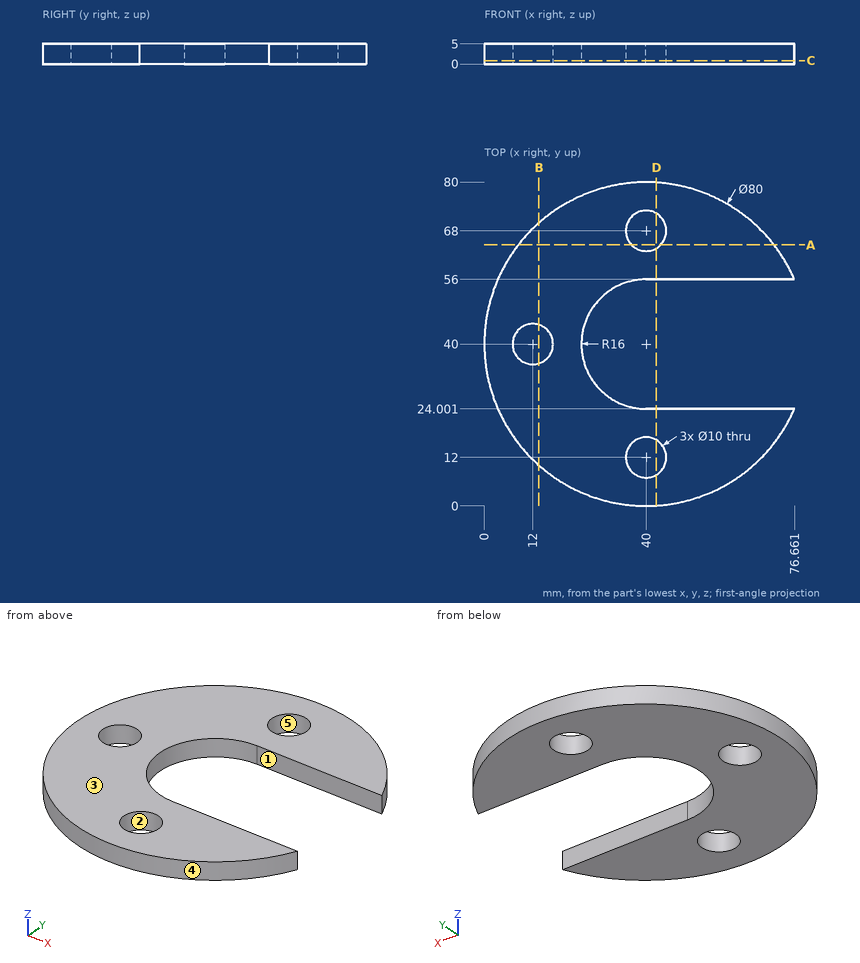
Design review of the part shown in the three views and the two pictorial views. Dimensions are in mm from the part's minimum x, y and z. A direction names the side the tool comes from. Give positions to 0.01 mm unless a question says otherwise; leave off trailing zeros. Write each loop counter-clockwise with the first axis right and the second up, starting at its lowest first coordinate (ties: lowest second). Pieces come first, ordered by that corner, then holes.
(1) Mouldability with a two-part tool opening along X and no side actions: class the marked faces 3, 4 and 5 as +X half, -X half, draft (parallel to the pull), parting line (faces both ways), or undercut.
Checked values:
face 3: draft
face 4: parting line
face 5: undercut
(2) Add section D-D (x = 42.5). Give the boundary of the cut face in (y, z).
Checked values:
outline: (0.08, 0) - (7.67, 0) - (7.67, 5) - (0.08, 5) - close; (16.33, 0) - (24, 0) - (24, 5) - (16.33, 5) - close; (56, 0) - (63.67, 0) - (63.67, 5) - (56, 5) - close; (72.33, 0) - (79.92, 0) - (79.92, 5) - (72.33, 5) - close
(3) Clearance check with flat-ended pins moving along their axes: pin 1 Ø1 at (x, z) = (62.5, 1.5) entering from +Y; pin 2 Ø1.5 at (x, z) = (62.5, 3.5) entering from -Y; pin 3 Ø3 at (y, z) = (9, 3) entering from +X (1 decimal). State where each tip first meets the part, or that it passes through.
Checked values:
pin 1: stops at y = 73.41
pin 2: stops at y = 6.43
pin 3: stops at x = 67
(4) Add section A-A (y = 64.5). Give the boundary of the cut face in (x, z).
Checked values:
outline: (8.38, 0) - (36.43, 0) - (36.43, 5) - (8.38, 5) - close; (43.57, 0) - (71.62, 0) - (71.62, 5) - (43.57, 5) - close
(5) Tool access review of the marked faces 1 and 2: name each direction out of +Z, -Z, +X, -X, +Y, -Y from which nothing blocks a thin tool from reaching the whole face with its end or side.
Checked values:
face 1: +Z, -Z, +X
face 2: +Z, -Z
(6) Wall thickness on line 1 along Y through (x, z) = (40, 2); line 2 along Y through (x, z) = (36.5, 3.7) (1 decimal); line 3 along X through (y, z) = (72.5, 2.9): over which ranges is each line inside the solid? List them lowest first.
Checked values:
line 1: y = 0 to 7, 17 to 24, 56 to 63, 73 to 80
line 2: y = 0.2 to 8.4, 15.6 to 24.4, 55.6 to 64.4, 71.6 to 79.8
line 3: x = 16.68 to 37.82, 42.18 to 63.32
(7) Add section B-B (x = 13.5). Give the boundary of the cut face in (y, z).
Checked values:
outline: (10.04, 0) - (35.23, 0) - (35.23, 5) - (10.04, 5) - close; (44.77, 0) - (69.96, 0) - (69.96, 5) - (44.77, 5) - close
(8) Add section C-C (z = 0.9). Give the boundary of the cut face in (x, y), and give its area (3 significant figures).
Checked values:
outline: (39.85, 24) arc R16 cw to (39.95, 56) - (76.66, 56) arc R40 ccw (long way) to (76.66, 24) - close; hole circle Ø10 at (12, 40); hole circle Ø10 at (40, 12); hole circle Ø10 at (40, 68)
area: 3,140 mm2
